```python
from build123d import *

# Parameters (mm, degrees)
SCHIZZO1_R                   = 1
ESTRUSIONE_ESTRUSIONE1_DEPTH = 2
RACCORDO2_R                  = 3
RACCORDO3_R                  = 3
RACCORDO4_R                  = 0.7
RACCORDO5_R                  = 0.7


with BuildPart() as part:
    # Schizzo1 → Estrusione-Estrusione1 (new body)
    with BuildSketch(Plane(origin=(0, 0, 0), x_dir=(0, 0, -1), z_dir=(1, 0, 0))):
        with BuildLine():
            add(Edge.make_bspline(
                [(-7.501010101, -10.3), (-10.845030199, -9.13986581), (-13.865102381, -7.304364218), (-17.601010101, -6.594005849)],
                knots=[0.271280726, 0.271280726, 0.271280726, 0.271280726, 0.852483684, 0.852483684, 0.852483684, 0.852483684], degree=3))
            add(Edge.make_bspline(
                [(-2.501010101, -11.3), (-4.308742426, -11.235865063), (-5.940164296, -10.841501107), (-7.501010101, -10.3)],
                knots=[0, 0, 0, 0, 0.271280726, 0.271280726, 0.271280726, 0.271280726], degree=3))
            Line((-2.501010101, -11.3), (1.498989899, -11.3))
            ThreePointArc((1.498989899, -11.3), (11.398989899, 0), (1.498989899, 11.3))
            Line((1.498989899, 11.3), (-2.501010101, 11.3))
            add(Edge.make_bspline(
                [(-2.501010101, 11.3), (-4.209338931, 11.338090952), (-5.850739142, 10.914740779), (-7.501010101, 10.3)],
                knots=[0, 0, 0, 0, 0.293888871, 0.293888871, 0.293888871, 0.293888871], degree=3))
            add(Edge.make_bspline(
                [(-7.501010101, 10.3), (-10.658273676, 9.123890914), (-13.848006436, 7.247243694), (-17.601010101, 6.561146452)],
                knots=[0.293888871, 0.293888871, 0.293888871, 0.293888871, 0.856150858, 0.856150858, 0.856150858, 0.856150858], degree=3))
            Line((-17.601010101, 6.561146452), (-17.601010101, 0))
            Line((-17.601010101, 0), (-17.601010101, -6.594005849))
        make_face()
        with Locations((5.5, -7)):
            Circle(SCHIZZO1_R, mode=Mode.SUBTRACT)
        with BuildLine():
            ThreePointArc((-12, 0), (-13, -1), (-14, 0))
            ThreePointArc((-14, 0), (-13, 1), (-12, 0))
        make_face(mode=Mode.SUBTRACT)
        Polygon((-10, -1.9), (-8.5, -1.9), (-8.5, 1.9), (-10, 1.9), (-10, 3.5), (-5.741010101, 3.5), (-5.741010101, 8.5), (2.258989899, 8.5), (2.258989899, 3.5), (9.198989899, 3.5), (9.198989899, -3.5), (2.258989899, -3.5), (2.258989899, -8.5), (-5.741010101, -8.5), (-5.741010101, -3.5), (-10, -3.5), align=None, mode=Mode.SUBTRACT)
        with Locations((5.5, 7)):
            Circle(SCHIZZO1_R, mode=Mode.SUBTRACT)
    extrude(amount=ESTRUSIONE_ESTRUSIONE1_DEPTH)

    # Raccordo2
    raccordo2_edges = [part.edges().sort_by_distance(p)[0] for p in [
        (1, -6.594005849, 17.601010101),
    ]]
    fillet(raccordo2_edges, radius=RACCORDO2_R)

    # Raccordo3
    raccordo3_edges = [part.edges().sort_by_distance(p)[0] for p in [
        (1, 6.561146452, 17.601010101),
    ]]
    fillet(raccordo3_edges, radius=RACCORDO3_R)

    # Raccordo4
    raccordo4_edges = [part.edges().sort_by_distance(p)[0] for p in [
        (1, -3.5, 5.741010101),
        (1, -8.5, 5.741010101),
        (1, -8.5, -2.258989899),
        (1, -3.5, -2.258989899),
        (1, -3.5, -9.198989899),
        (1, 3.5, -9.198989899),
        (1, 3.5, -2.258989899),
        (1, 8.5, -2.258989899),
        (1, 8.5, 5.741010101),
        (1, 3.5, 5.741010101),
    ]]
    fillet(raccordo4_edges, radius=RACCORDO4_R)

    # Raccordo5
    raccordo5_edges = [part.edges().sort_by_distance(p)[0] for p in [
        (1, 1.9, 8.5),
        (1, -1.9, 8.5),
    ]]
    fillet(raccordo5_edges, radius=RACCORDO5_R)


solid = part.part
```
Design review of the part built by this model. Coordinates are the model's own, in mm. A direction names the side the tool comes from. Coordinates: 2 decimals unless noted, no trailing zeros. Order: outer loops, then holes, each group sorted by start corner. A loop starts at its lowest first (then second) coordinate and runs counter-clockwise, first axis right, second up. Notation, with made-up numbers: (85.25, 19.25) -> (109.25, 19.25) arc R19 cw to (109.25, 48.25) -> close; hole circle Ø10 at (55.25, 4). An arc over 180 degrees is marked (long way). One line per item, written item: value. Start each with the question number.
Q1. Tool access review of faces 4 (the flat face through (1, 0, 17.601)), 5 (the flat face through (1, 3.5, -6)): name each direction out of +Z, -Z, +X, -X, +Y, -Y from which nothing blocks a thin tool from reaching the whole face with its end or side.
Q2. For probe 1 along Y at (x, z) = (1.2, -1.25); probe 2 along Z at (x, y) = (0.5, 0.25); probe 3 along Z at (x, y) = (1.6, 4.5), list the stretches that pass through material, from the lowest coordinate up.
Q3. Take a section at B-B, the plane x = 1.5. Give the number of separate pieces and of enclosed holes in the cut face, then the cut area to 3 significant figures.
Q4. Insertion check: pin 1 Ø1 at (x, y) = (1, 6) entering from -Z; pin 2 Ø1 at (x, z) = (1, -6.5) entering from +Y; pin 3 Ø1 at (x, y) = (1.5, -6) entering from +Z. Each pin has a flat end and moves straight along its axis. Give the tip position at first contact, or say it passes through.
Q5. Mouldability with a two-part tool opening along Y and no side actions: class faces 1 (the flat face through (1, -11.3, 1)), 2 (the flat face through (1, -1.9, 9.6)), 3 (the flat face through (2, -5, 6)) as pulls with the +Y half, pulls with the -Y half, needs draft (parallel to the pull), parting line crosses it, or undercut.
Q6. Take a section at A-A, the plane z = -5.5. State the section outline as (x, y) points, then the cut area to 3 significant figures.
Values follow:
1. face 4: +Z, +X, -X, +Y, -Y
1. face 5: +X, -X
2. probe 1: y = -11.3 to -8.5, 8.5 to 11.3
2. probe 2: z = -11.4 to -9.2, 8.5 to 12.03, 13.97 to 17.6
2. probe 3: z = -10.47 to -2.26, 5.74 to 17.59
3. separate pieces: 1
3. enclosed holes: 4
3. area: 317 mm2
4. pin 1: stops at z = -9.98
4. pin 2: stops at y = 9.69
4. pin 3: stops at z = 17.33
5. face 1: pulls with the -Y half
5. face 2: undercut
5. face 3: needs draft
6. outline: (0, -9.98) -> (2, -9.98) -> (2, -8) -> (0, -8) -> close; (0, -6) -> (2, -6) -> (2, -3.5) -> (0, -3.5) -> close; (0, 3.5) -> (2, 3.5) -> (2, 6) -> (0, 6) -> close; (0, 8) -> (2, 8) -> (2, 9.98) -> (0, 9.98) -> close
6. area: 17.9 mm2
